```python
from build123d import *

# Parameters (mm, degrees)
BOSS_EXTRUDE1_DEPTH = 60
SKETCH2_R           = 1.6
CUT_EXTRUDE1_DEPTH  = 20
SKETCH4_W           = 2
SKETCH4_H           = 4
CUT_EXTRUDE2_DEPTH  = 10
BOSS_EXTRUDE2_DEPTH = 9


with BuildPart() as part:
    # Sketch1 → Boss-Extrude1 (new body)
    with BuildSketch(Plane(origin=(0, 0, 0), x_dir=(1, 0, 0), z_dir=(0, 1, 0))):
        with BuildLine():
            Line((40, 0), (0, 0))
            Line((0, 0), (8.550503583, -23.49231552))
            add(Edge.make_bspline(
                [(8.550503583, -23.49231552), (9.187650747, -24.984982914), (10.869033495, -26.695868857), (13.579943454, -28.275526589), (21.375498678, -32.059284682), (31.165356306, -32.945912064), (37.204636828, -29.076990777)],
                knots=[0, 0, 0, 0, 0.15219933, 0.226855665, 0.301953476, 0.995167611, 0.995167611, 0.995167611, 0.995167611], degree=3))
            add(Edge.make_bspline(
                [(37.204636828, -29.076990777), (37.246736594, -29.050020564), (37.288700602, -29.022823469), (37.330527165, -28.995398615)],
                knots=[0.995167611, 0.995167611, 0.995167611, 0.995167611, 1, 1, 1, 1], degree=3))
            ThreePointArc((37.330527165, -28.995398615), (39.290627696, -26.837555683), (40, -24.01))
            Line((40, -24.01), (40, 0))
        make_face()
    extrude(amount=BOSS_EXTRUDE1_DEPTH)

    # Sketch2 → Cut-Extrude1 (cut)
    with BuildSketch(Plane(origin=(0, 0, 0), x_dir=(-1, 0, 0), z_dir=(0, 0, -1))):
        with Locations((-34, 36)):
            Circle(SKETCH2_R)
        with Locations((-34, 24)):
            Circle(SKETCH2_R)
    extrude(amount=-CUT_EXTRUDE1_DEPTH, mode=Mode.SUBTRACT)

    # Sketch4 → Cut-Extrude2 (cut)
    with BuildSketch(Plane(origin=(40, 0, 0), x_dir=(0, 0, -1), z_dir=(1, 0, 0))):
        with Locations((-15, 24)):
            Rectangle(SKETCH4_W, SKETCH4_H)
        with Locations((-15, 36)):
            Rectangle(SKETCH4_W, SKETCH4_H)
    extrude(amount=-CUT_EXTRUDE2_DEPTH, mode=Mode.SUBTRACT)

    # Sketch5 → Boss-Extrude2 (add)
    with BuildSketch(Plane(origin=(0, 0, 0), x_dir=(-1, 0, 0), z_dir=(0, 0, -1))):
        Polygon((-31.369100365, 42.428714266), (-32.760831375, 52.331394953), (-22.858150687, 53.723125963), (-21.466419678, 43.820445275), align=None)
        Polygon((-31.369100365, 17.571285734), (-32.760831375, 7.668605047), (-22.858150687, 6.276874037), (-21.466419678, 16.179554725), align=None)
    extrude(amount=BOSS_EXTRUDE2_DEPTH)

    # Sketch6 → Revolve1 (revolve)
    with BuildSketch(Plane(origin=(34, 0, 0), x_dir=(0, 0, -1), z_dir=(1, 0, 0))):
        Polygon((0, 37.6), (2, 37.6), (0, 38.6), align=None)
    revolve(axis=Axis((34, 36, 0), (0, 0, -1)))

    # Sketch7 → Revolve2 (revolve)
    with BuildSketch(Plane(origin=(34, 0, 0), x_dir=(0, 0, -1), z_dir=(1, 0, 0))):
        Polygon((0, 25.6), (2, 25.6), (0, 26.6), align=None)
    revolve(axis=Axis((34, 24, 0), (0, 0, -1)))


solid = part.part
```
Model file for the job. Use its own axes, mm. A direction names the side the tool comes from. Coordinates: 2 decimals unless noted, no trailing zeros. Write each loop counter-clockwise with the first axis right and the second up, starting at its lowest first coordinate (ties: lowest second). Pieces come first, ordered by that corner, then holes. Notation, with made-up numbers: (61.5, 81.25) - (79.5, 81.25) arc R6 ccw to (79.5, 92.25) - close; hole circle Ø11 at (61.5, 38.25). An arc over 180 degrees is marked (long way). Use a Markdown table: item, result. Add a question column.
Item 1: Band-saw the part on B-B, the plane z = 10.5. Write the cut outline in (x, y), and give its area (3 significant figures).
Item 2: Drill centre lines: line 1 along Y through (x, z) = (34, 4.5); line 2 along Z through (x, y) = (27, 51); line 3 along Z through (x, y) = (23, 28.5). Where is each one in solid material? Low to high.
Item 3: 3-axis set-ups, long thin cutter, end or side, ignore diameter. For faces 1 (the face through (32.055, 47.311, -4.437)), 2 (the face through (22.17, 48.84, -4.44)), 3 (the face through (22.17, 11.16, -4.44)), 4 (the face through (34, 36, 20)): which of +Z, -Z, +X, -X, +Y, -Y reach the whole face in a straight line?
Item 4: Band-saw the part on C-C, the plane z = 4. Write the cut outline in (x, y), and give its area (3 significant figures).
Item 5: Band-saw the part on A-A, the plane z = -3.5. Write the cut outline in (x, y).
Item 6: Two-plate mould, pull along Y, no slides. Class faces 5 (the face through (27, 48, -9)), 6 (the face through (35, 34, 15)), 7 (the face through (28, 7, -4)): pulls with the +Y half, pulls with the -Y half, needs draft (parallel to the pull), parting line crosses it, or undercut.
Item 7: Drop flat-ended pins along their axis: pin 1 (4 mm diameter, centred on x = 34, y = 36, fed in from +Z); pin 2 (2 mm diameter, centred on y = 36, z = 14.5, fed in from +X); pin 3 (3.5 mm diameter, centred on x = 34, y = 24, fed in from -Z); pin 4 (5 mm diameter, centred on x = 34, y = 24, fed in from +Z). Give the stop position or say it passes through.
A:
| question | item | result |
|---|---|---|
| 1 | outline | (3.82, 0) - (40, 0) - (40, 60) - (3.82, 60) - close; hole circle Ø3.2 at (34, 24); hole circle Ø3.2 at (34, 36) |
| 1 | area | 2,150 mm² |
| 2 | line 1 | y = 0 to 22.4, 25.6 to 34.4, 37.6 to 60 |
| 2 | line 2 | z = -9 to 31.71 |
| 2 | line 3 | z = 0 to 31.37 |
| 3 | face 1 | -Z, +X |
| 3 | face 2 | -Z, -X, +Y |
| 3 | face 3 | -Z, -X, -Y |
| 3 | face 4 | -Z |
| 4 | outline | (1.46, 0) - (40, 0) - (40, 60) - (1.46, 60) - close; hole circle Ø3.2 at (34, 24); hole circle Ø3.2 at (34, 36) |
| 4 | area | 2,300 mm² |
| 5 | outline | (21.47, 16.18) - (22.86, 6.28) - (32.76, 7.67) - (31.37, 17.57) - close; (21.47, 43.82) - (31.37, 42.43) - (32.76, 52.33) - (22.86, 53.72) - close |
| 6 | face 5 | needs draft |
| 6 | face 6 | undercut |
| 6 | face 7 | pulls with the -Y half |
| 7 | pin 1 | stops at z = 31.2 |
| 7 | pin 2 | stops at x = 40 |
| 7 | pin 3 | stops at z = -2 |
| 7 | pin 4 | stops at z = 31.3 |
